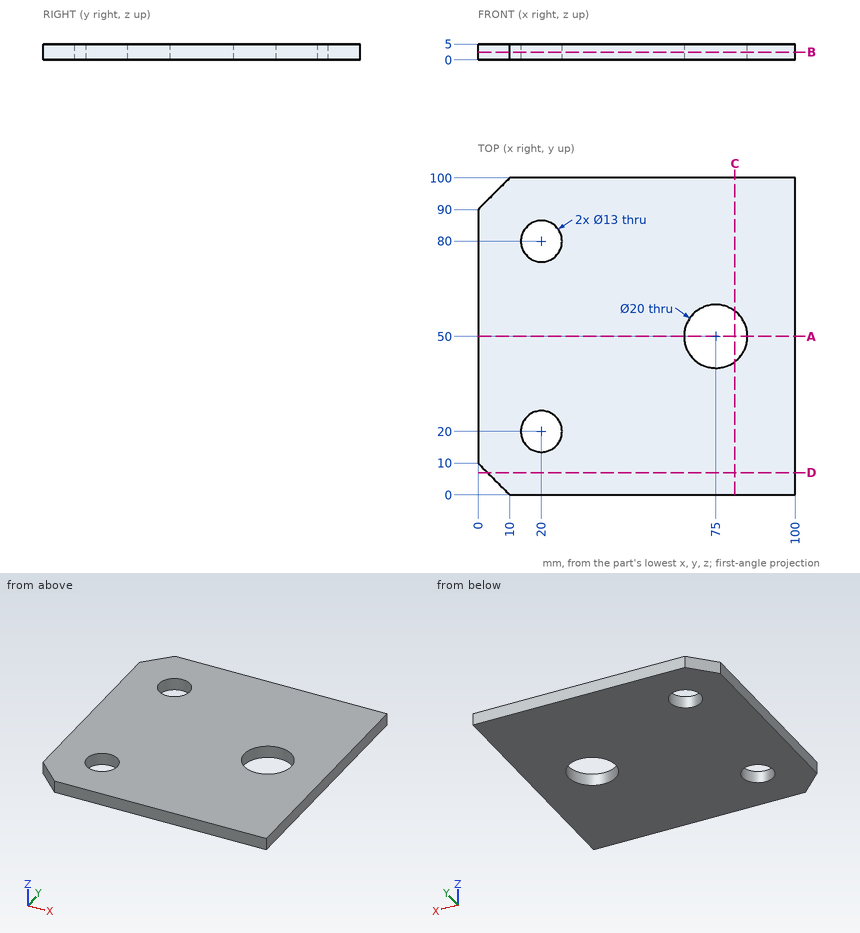
Here's the drawing with two shaded views (mm, measured from the low corner). I have some questions. Give positions to 0.01 mm unless a question says otherwise; leave off trailing zeros. Loops run counter-clockwise (first coordinate to the right, second up) from the corner with the lowest first, then second, coordinate; pieces in that order, holes last. Notation, with made-up numbers: (76, -38) - (114, -38) arc R17 ccw to (114, -16) - close; hole circle Ø6 at (53.5, -3.75). An arc over 180 degrees is marked (long way). Return JSON: item names as keys, results as strings.
1. I want a section at C-C on x = 81. Please give me the cut outline in (y, z).
Output values:
{"outline": "(0, 0) - (42, 0) - (42, 5) - (0, 5) - close; (58, 0) - (100, 0) - (100, 5) - (58, 5) - close"}
2. I want a section at D-D on y = 7. Please give me the cut outline in (x, z), and give its area (3 significant figures).
Output values:
{"outline": "(3, 0) - (100, 0) - (100, 5) - (3, 5) - close", "area": "485 mm²"}
3. I'm going to push a flat-ended pin straight in: pin 1 Ø11.5 at (x, y) = (20, 20) entering from -Z. Where does the tip first touch, or does it pass through?
Output values:
{"pin 1": "passes through"}
4. If I drill on line 1 (Y direction, x = 20, z = 1.2); line 2 (Y direction, x = 24.5, z = 2.75); line 3 (Y direction, x = 75, z = 2.85), over which ranges is the centre line in solid material (lowest first)?
Output values:
{"line 1": "y = 0 to 13.5, 26.5 to 73.5, 86.5 to 100", "line 2": "y = 0 to 15.31, 24.69 to 75.31, 84.69 to 100", "line 3": "y = 0 to 40, 60 to 100"}
5. I want a section at B-B on z = 2.45. Please give me the cut outline in (x, y), and give its area (3 significant figures).
Output values:
{"outline": "(0, 10) - (10, 0) - (100, 0) - (100, 100) - (10, 100) - (0, 90) - close; hole circle Ø13 at (20, 20); hole circle Ø13 at (20, 80); hole circle Ø20 at (75, 50)", "area": "9,320 mm²"}
6. I want a section at A-A on y = 50. Please give me the cut outline in (x, z).
Output values:
{"outline": "(0, 0) - (65, 0) - (65, 5) - (0, 5) - close; (85, 0) - (100, 0) - (100, 5) - (85, 5) - close"}
